```python
from build123d import *

# Parameters (mm, degrees)
BOSS_EXTRUDE1_DEPTH      = 80
BOSS_EXTRUDE1_DEPTH_BACK = 80
SKETCH1_R                = 9


with BuildPart() as part:
    # Sketch1 → Boss-Extrude1 (new, two sides: drawn at the far end of the back side and taken through both)
    with BuildSketch(Plane(origin=(0, 0, 0), x_dir=(0, 0, -1), z_dir=(1, 0, 0)).offset(-BOSS_EXTRUDE1_DEPTH_BACK)):
        with BuildLine():
            Line((-10, 125), (-10, -120))
            Line((-10, -120), (-9, -120))
            Line((-9, -120), (-9, 120.641101056))
            ThreePointArc((-9, 120.641101056), (9.746794345, 127.236067977), (-10, 125))
        make_face()
        with Locations((0, 125)):
            Circle(SKETCH1_R, mode=Mode.SUBTRACT)
    extrude(amount=BOSS_EXTRUDE1_DEPTH + BOSS_EXTRUDE1_DEPTH_BACK)


solid = part.part
```
Here's how the part is built. I have some questions about the finished solid (model axes, mm). Coordinates: 2 decimals unless noted, no trailing zeros. Write each loop counter-clockwise with the first axis right and the second up, starting at its lowest first coordinate (ties: lowest second). Pieces come first, ordered by that corner, then holes. Notation, with made-up numbers: (88.5, -1) - (110.5, -1) arc R23 ccw to (110.5, 15) - close; hole circle Ø9 at (-18, 49.25). An arc over 180 degrees is marked (long way). One line per item, written item: value.
1) Suppose I cut it at C-C on y = 95. Write out the boundary of the cut face in (x, z), and give its area (3 significant figures).
Model answer:
outline: (-80, 9) - (80, 9) - (80, 10) - (-80, 10) - close
area: 160 mm²
2) We'd pull the mould along Y, two halves only. Please class faces 1 (the flat face through (80, 17.5, 9.7)), 2 (the cylindrical face through (-1.12, 133.923, 1.172)): pulls with the +Y half, pulls with the -Y half, needs draft (parallel to the pull), parting line crosses it, or undercut.
Model answer:
face 1: needs draft
face 2: undercut
3) I'm going to push flat-ended pins straight in: P1, Ø1.5, axis at x = -16, z = 1, coming from the -Y side; P2, Ø4, axis at x = -48, z = 3.5, coming from the +Y side; P3, Ø12, axis at x = -56, y = 19, coming from the -Z side; P4, Ø1, axis at y = 78.5, z = 8, coming from the +X side. Where does each tip first touch, or does it pass through?
Model answer:
P1: stops at y = 115
P2: stops at y = 134.89
P3: stops at z = 9
P4: passes through
4) I need wall thicknesses on line 1 along Y through (x, z) = (48, -0.75); line 2 along Y through (x, z) = (13, 1); line 3 along Z through (x, y) = (-28, -68). Which ranges of each line are inside material? Lowest first, please.
Model answer:
line 1: y = 115.03 to 116.03, 133.97 to 134.97
line 2: y = 115.05 to 116.06, 133.94 to 134.95
line 3: z = 9 to 10
5) Suppose I cut it at B-B on x = 67. Write out the boundary of the cut face in (y, z), and give its area (3 significant figures).
Model answer:
outline: (-120, 9) - (120.64, 9) arc R10 ccw (long way) to (125, 10) - (-120, 10) - close; hole circle Ø18 at (125, 0)
area: 302 mm²
6) Suppose I cut it at A-A on z = 0. Write out the boundary of the cut face in (x, y).
Model answer:
outline: (-80, 115) - (80, 115) - (80, 116) - (-80, 116) - close; (-80, 134) - (80, 134) - (80, 135) - (-80, 135) - close
